from build123d import *

# Parameters (mm, degrees)
SKIZZE1_W                       = 48
SKIZZE1_H                       = 44
AUFSATZ_LINEAR_AUSTRAGEN1_DEPTH = 3
SKIZZE2_W                       = 48
SKIZZE2_H                       = 4
AUFSATZ_LINEAR_AUSTRAGEN2_DEPTH = 44
SKIZZE3_R                       = 11.5
SKIZZE3_R_2                     = 1.6
SCHNITT_LINEAR_AUSTRAGEN1_DEPTH = 67.219332525
SKIZZE5_W                       = 2
SKIZZE5_H                       = 40
AUFSATZ_LINEAR_AUSTRAGEN3_DEPTH = 5
FASE2_SIZE                      = 5
FASE3_SIZE                      = 4
AUFSATZ_LINEAR_AUSTRAGEN4_DEPTH = 2
FASE4_SIZE                      = 2
SKIZZE8_R                       = 1.25
SCHNITT_LINEAR_AUSTRAGEN2_DEPTH = 71.689461732


with BuildPart() as part:
    # Skizze1 → Aufsatz-Linear austragen1 (new body)
    with BuildSketch(Plane(origin=(0, 0, 0), x_dir=(1, 0, 0), z_dir=(0, 1, 0))):
        Rectangle(SKIZZE1_W, SKIZZE1_H)
    extrude(amount=AUFSATZ_LINEAR_AUSTRAGEN1_DEPTH)

    # Skizze2 → Aufsatz-Linear austragen2 (add)
    with BuildSketch(Plane(origin=(0, 3, 0), x_dir=(1, 0, 0), z_dir=(0, 1, 0))):
        with Locations((0, 20)):
            Rectangle(SKIZZE2_W, SKIZZE2_H)
    extrude(amount=AUFSATZ_LINEAR_AUSTRAGEN2_DEPTH)

    # Skizze3 → Schnitt-Linear austragen1 (cut, through all)
    with BuildSketch(Plane.XY.offset(-18)):
        with Locations((0, 25)):
            Circle(SKIZZE3_R)
        with Locations((-15.55, 40.55)):
            Circle(SKIZZE3_R_2)
        with Locations((15.55, 40.55)):
            Circle(SKIZZE3_R_2)
        with Locations((15.55, 9.45)):
            Circle(SKIZZE3_R_2)
        with Locations((-15.55, 9.45)):
            Circle(SKIZZE3_R_2)
    extrude(amount=-SCHNITT_LINEAR_AUSTRAGEN1_DEPTH, mode=Mode.SUBTRACT)

    # Skizze5 → Aufsatz-Linear austragen3 (add)
    with BuildSketch(Plane(origin=(0, 3, 0), x_dir=(1, 0, 0), z_dir=(0, 1, 0))):
        with Locations((-23, -2)):
            Rectangle(SKIZZE5_W, SKIZZE5_H)
        with Locations((23, -2)):
            Rectangle(SKIZZE5_W, SKIZZE5_H)
    extrude(amount=AUFSATZ_LINEAR_AUSTRAGEN3_DEPTH)

    # Fase2
    fase2_edges = [part.edges().sort_by_distance(p)[0] for p in [
        (23, 8, -18),
        (-23, 8, 22),
        (-23, 8, -18),
        (23, 8, 22),
    ]]
    chamfer(fase2_edges, length=FASE2_SIZE)

    # Fase3
    fase3_edges = [part.edges().sort_by_distance(p)[0] for p in [
        (-24, 47, -20),
        (24, 47, -20),
    ]]
    chamfer(fase3_edges, length=FASE3_SIZE)

    # Skizze7 → Aufsatz-Linear austragen4 (add)
    with BuildSketch(Plane.XZ):
        Polygon((-1.75, 22), (1.75, 22), (1.75, 17.95), (1, 17.2), (-1, 17.2), (-1.75, 17.95), align=None)
    extrude(amount=AUFSATZ_LINEAR_AUSTRAGEN4_DEPTH)

    # Fase4
    fase4_edges = [part.edges().sort_by_distance(p)[0] for p in [
        (0, -2, 17.2),
        (0, -2, 22),
    ]]
    chamfer(fase4_edges, length=FASE4_SIZE - 0.0001)  # a hair under: the kernel refuses the full size

    # Skizze8 → Schnitt-Linear austragen2 (cut, through all)
    with BuildSketch(Plane.ZY.offset(24)):
        with Locations((16.83, 4.6)):
            Circle(SKIZZE8_R)
        with Locations((10.33, 4.6)):
            Circle(SKIZZE8_R)
    extrude(amount=-SCHNITT_LINEAR_AUSTRAGEN2_DEPTH, mode=Mode.SUBTRACT)


solid = part.part
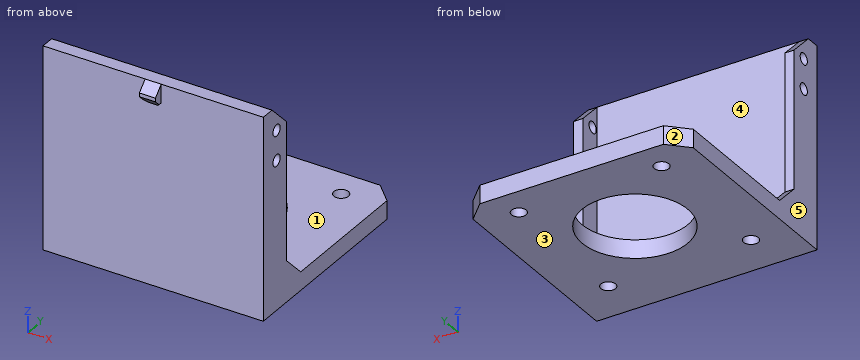
Verification items for the finished model (mm, model axes). Face numbers are marked on the shaded views. A direction names the side the tool comes from. Give positions to 0.01 mm unless a question says otherwise; leave off trailing zeros. Write each loop counter-clockwise with the first axis right and the second up, starting at its lowest first coordinate (ties: lowest second). Pieces come first, ordered by that corner, then holes.
(1) Cross-section at B-B (y = 25). Enter the section's corners in (x, z).
(2) Mould release check, pull along X, two halves, no side actions. Record for the marked faces 3, 4 and 5: +X half, -X half, draft (parallel to the pull), parting line (faces both ways), or undercut.
(3) Cross-section at C-C (z = -14). Enter the section's corners in (x, y), plus the area to 3 significant figures.
(4) Material ranges on line 1 (Y direction, x = -15.55, z = -20.05); line 2 (X direction, y = 7.5, z = 7.5); line 3 (Y direction, x = 0, z = -19), recorded low to high.
(5) Access from +Z, -Z, +X, -X, +Y, -Y to the whole of each face (thin tool, end or side, straight path). Record for the marked faces 1 and 2.
(6) Cross-section at A-A (x = 15.55). Enter the section's corners in (y, z).
(7) Gauge pin test, flat ends, axial feed: pin 1 (2 mm diameter, centred on x = 15.5, z = -12.5, fed in from +Y); pin 2 (14 mm diameter, centred on x = 0, y = 25, fed in from +Z); pin 3 (22 mm diameter, centred on x = 0.5, y = 30, fed in from +Z); pin 4 (2 mm diameter, centred on x = 22.5, z = 4.5, fed in from +Y). Record the tip position at first contact, or that the pin passes through.
Worked out:
1. outline: (-24, -22) - (-11.5, -22) - (-11.5, -18) - (-24, -18) - close; (11.5, -22) - (24, -22) - (24, -18) - (11.5, -18) - close
2. face 3: draft
2. face 4: undercut
2. face 5: -X half
3. outline: (-24, 0) - (24, 0) - (24, 9) - (22, 9) - (22, 3) - (-22, 3) - (-22, 9) - (-24, 9) - close
3. area: 168 mm2
4. line 1: y = 0 to 7.85, 11.05 to 38.95, 42.15 to 47
4. line 2: x = -24 to -22, 22 to 24
4. line 3: y = 0 to 13.5, 36.5 to 47
5. face 1: +Z, +Y
5. face 2: +Z, -Z, -X, +Y
6. outline: (0, -22) - (7.85, -22) - (7.85, -18) - (3, -18) - (3, 22) - (0, 22) - close; (11.05, -22) - (38.95, -22) - (38.95, -18) - (11.05, -18) - close; (42.15, -22) - (47, -22) - (47, -18) - (42.15, -18) - close
7. pin 1: stops at y = 3
7. pin 2: passes through
7. pin 3: stops at z = -18
7. pin 4: stops at y = 8
